from build123d import *

# Parameters (mm, degrees)
SKETCH_1_W               = 120
SKETCH_1_H               = 50
EXTRUDE_2_DEPTH          = 2.5
SKETCH_1_3_R             = 1.75
SKETCH_1_3_W             = 68
SKETCH_1_3_H             = 31
CUT_EXTRUDE_1_DEPTH      = 66.296266207
EXTRUDE_START            = -60
EXTRUDE_3_DEPTH          = 120
EXTRUDE_3_2_DEPTH        = 2.5
EXTRUDE_START_2          = 57.5
EXTRUDE_3_3_DEPTH        = 2.5
CUT_EXTRUDE_2_DEPTH      = 129.109700543
CUT_EXTRUDE_2_DEPTH_BACK = 129.109700543
EXTRUDE_4_DEPTH          = 120
EXTRUDE_5_REACH          = 77.063
EXTRUDE_6_REACH          = 77.063
SKETCH_7_R               = 2.5
CUT_EXTRUDE_3_DEPTH      = 5
SKETCH_8_R               = 1.75
CUT_EXTRUDE_4_DEPTH      = 5
EXTRUDE_8_DEPTH          = 120
SKETCH_10_W              = 3.2
SKETCH_10_H              = 2.2
CUT_EXTRUDE_5_DEPTH      = 10


# Read off the part's stored shape, not the designer's step: 凸台-拉伸3
with BuildPart() as part:
    # 草图1 → 凸台-拉伸2 (new, along a direction that is not the sketch's normal)
    with BuildSketch(Plane(origin=(0, 0, 0), x_dir=(1, 0, 0), z_dir=(0, 1, 0))):
        Rectangle(SKETCH_1_W, SKETCH_1_H)
    extrude(amount=EXTRUDE_2_DEPTH, dir=(0, 0.9659258262890672, 0.2588190451025249))

    # 草图1<3> → 切除-拉伸1 (cut, through all)
    with BuildSketch(Plane(origin=(0, 0, 0), x_dir=(1, 0, 0), z_dir=(0, 1, 0))):
        with Locations(Location((-45.5, 16.5, 0), (0, 0, 270))):
            Circle(SKETCH_1_3_R)
        with Locations(Location((-45.5, -16.5, 0), (0, 0, 270))):
            Circle(SKETCH_1_3_R)
        Rectangle(SKETCH_1_3_W, SKETCH_1_3_H)
        with BuildLine():
            Line((41.5, 18.25), (40.5, 18.25))
            ThreePointArc((40.5, 18.25), (38.75, 16.5), (40.5, 14.75))
            Line((40.5, 14.75), (41.5, 14.75))
            ThreePointArc((41.5, 14.75), (43.25, 16.5), (41.5, 18.25))
        make_face()
        with BuildLine():
            Line((41.5, -18.25), (40.5, -18.25))
            ThreePointArc((40.5, -18.25), (38.75, -16.5), (40.5, -14.75))
            Line((40.5, -14.75), (41.5, -14.75))
            ThreePointArc((41.5, -14.75), (43.25, -16.5), (41.5, -18.25))
        make_face()
    extrude(amount=CUT_EXTRUDE_1_DEPTH, mode=Mode.SUBTRACT)

    # 凸台-拉伸3 outline → 凸台-拉伸3 (add)
    with BuildSketch(Plane.YZ.offset(EXTRUDE_START)):
        Polygon((-10.306305876, -25.173375885), (-9.659258263, -27.588190451), (0, -25), (0, -22.411809549), align=None)
        Polygon((-25.188400969, 30.367359126), (-24.541353356, 27.952544561), (0, 34.528380374), (0, 37.116570825), align=None)
    extrude(amount=EXTRUDE_3_DEPTH)

    # Extrude 3 2 outline → Extrude 3 2 (add)
    with BuildSketch(Plane.YZ.offset(EXTRUDE_START)):
        Polygon((-24.541353356, 27.952544561), (-10.306305876, -25.173375885), (0, -22.411809549), (0, 34.528380374), align=None)
    extrude(amount=EXTRUDE_3_2_DEPTH)

    # Extrude 3 3 outline → Extrude 3 3 (add)
    with BuildSketch(Plane.YZ.offset(EXTRUDE_START_2)):
        Polygon((-24.541353356, 27.952544561), (-10.306305876, -25.173375885), (0, -22.411809549), (0, 34.528380374), align=None)
    extrude(amount=EXTRUDE_3_3_DEPTH)

    # 草图4 → 切除-拉伸2 (cut, two sides: drawn at the far end of the back side and taken through both)
    with BuildSketch(Plane.ZY.offset(60).offset(-CUT_EXTRUDE_2_DEPTH_BACK)):
        Polygon((25.647047613, 2.414814566), (36.951962095, -0.61432814), (37.116570825, 0), align=None)
    extrude(amount=CUT_EXTRUDE_2_DEPTH + CUT_EXTRUDE_2_DEPTH_BACK, mode=Mode.SUBTRACT)

    # 草图5 → 凸台-拉伸4 (add)
    with BuildSketch(Plane.ZY.offset(60)):
        Polygon((25.647047613, 2.414814566), (36.951962095, -0.61432814), (36.304914483, -3.029142706), (25, 0), align=None)
    extrude(amount=-EXTRUDE_4_DEPTH)

    # 凸台-拉伸5: up to this plane
    extrude_5_end = Plane(origin=(0, 0, 0), z_dir=(0, 1, 0))
    # 草图6 → 凸台-拉伸5 (add, up to the surface)
    with BuildSketch(Plane(origin=(0, -15.909258263, -4.262872904), x_dir=(1, 0, 0), z_dir=(0, -0.9659258262890672, -0.25881904510252496)), mode=Mode.PRIVATE) as extrude_5_sk1:
        with BuildLine():
            Line((-60, -24.148145657), (-52, -24.148145657))
            Line((-52, -24.148145657), (-52, -20.148145657))
            ThreePointArc((-52, -20.148145657), (-53.171572875, -17.319718532), (-56, -16.148145657))
            Line((-56, -16.148145657), (-60, -16.148145657))
            Line((-60, -16.148145657), (-60, -24.148145657))
        make_face()
    extrude_5_tool1 = split(extrude(extrude_5_sk1.sketch, amount=-EXTRUDE_5_REACH, mode=Mode.PRIVATE), bisect_by=extrude_5_end, keep=Keep.BOTH, mode=Mode.PRIVATE)
    add(extrude_5_tool1.solids().sort_by_distance((-56.176115, -10.648952, -23.894601))[0])
    # 草图6 → 凸台-拉伸5 (add, up to the surface)
    with BuildSketch(Plane(origin=(0, -15.909258263, -4.262872904), x_dir=(1, 0, 0), z_dir=(0, -0.9659258262890672, -0.25881904510252496)), mode=Mode.PRIVATE) as extrude_5_sk2:
        with BuildLine():
            Line((60, -24.148145657), (52, -24.148145657))
            Line((52, -24.148145657), (52, -20.148145657))
            ThreePointArc((52, -20.148145657), (53.171572875, -17.319718532), (56, -16.148145657))
            Line((56, -16.148145657), (60, -16.148145657))
            Line((60, -16.148145657), (60, -24.148145657))
        make_face()
    extrude_5_tool2 = split(extrude(extrude_5_sk2.sketch, amount=-EXTRUDE_5_REACH, mode=Mode.PRIVATE), bisect_by=extrude_5_end, keep=Keep.BOTH, mode=Mode.PRIVATE)
    add(extrude_5_tool2.solids().sort_by_distance((56.176115, -10.648952, -23.894601))[0])

    # 草图6<4> → 凸台-拉伸6 (add, up to next)
    with BuildSketch(Plane(origin=(0, -15.909258263, -4.262872904), x_dir=(1, 0, 0), z_dir=(0, -0.9659258262890672, -0.25881904510252496)), mode=Mode.PRIVATE) as extrude_6_sk1:
        with BuildLine():
            Line((-60, 35.851854343), (-52, 35.851854343))
            Line((-52, 35.851854343), (-52, 31.851854343))
            ThreePointArc((-52, 31.851854343), (-53.171572875, 29.023427218), (-56, 27.851854343))
            Line((-56, 27.851854343), (-60, 27.851854343))
            Line((-60, 27.851854343), (-60, 35.851854343))
        make_face()
    extrude_6_tool1 = extrude(extrude_6_sk1.sketch, amount=-EXTRUDE_6_REACH, mode=Mode.PRIVATE) - part.part
    # 草图6<4> → 凸台-拉伸6 (add, up to next)
    with BuildSketch(Plane(origin=(0, -15.909258263, -4.262872904), x_dir=(1, 0, 0), z_dir=(0, -0.9659258262890672, -0.25881904510252496)), mode=Mode.PRIVATE) as extrude_6_sk2:
        with BuildLine():
            Line((60, 35.851854343), (52, 35.851854343))
            Line((52, 35.851854343), (52, 31.851854343))
            ThreePointArc((52, 31.851854343), (53.171572875, 29.023427218), (56, 27.851854343))
            Line((56, 27.851854343), (60, 27.851854343))
            Line((60, 27.851854343), (60, 35.851854343))
        make_face()
    extrude_6_tool2 = extrude(extrude_6_sk2.sketch, amount=-EXTRUDE_6_REACH, mode=Mode.PRIVATE) - part.part
    add(extrude_6_tool1.solids().sort_by_distance((-56.176115, -24.198707, 26.67377))[0])
    add(extrude_6_tool2.solids().sort_by_distance((56.176115, -24.198707, 26.67377))[0])

    # 草图7 → 切除-拉伸3 (cut)
    with BuildSketch(Plane(origin=(0, -15.909258263, -4.262872904), x_dir=(1, 0, 0), z_dir=(0, -0.9659258262890672, -0.25881904510252496))):
        with Locations(Location((-56, 31.851854343, 0), (0, 0, 270))):
            Circle(SKETCH_7_R)
        with Locations(Location((-56, -20.148145657, 0), (0, 0, 270))):
            Circle(SKETCH_7_R)
        with Locations(Location((56, -20.148145657, 0), (0, 0, 270))):
            Circle(SKETCH_7_R)
        with Locations(Location((56, 31.851854343, 0), (0, 0, 270))):
            Circle(SKETCH_7_R)
    extrude(amount=-CUT_EXTRUDE_3_DEPTH, mode=Mode.SUBTRACT)

    # 草图8 → 切除-拉伸4 (cut)
    with BuildSketch(Plane(origin=(0, -11.079629131, -2.968777678), x_dir=(1, 0, 0), z_dir=(0, -0.9659258262890672, -0.25881904510252496))):
        with Locations(Location((-56, 31.851854343, 0), (0, 0, 270))):
            Circle(SKETCH_8_R)
        with Locations(Location((-56, -20.148145657, 0), (0, 0, 270))):
            Circle(SKETCH_8_R)
        with Locations(Location((56, -20.148145657, 0), (0, 0, 270))):
            Circle(SKETCH_8_R)
        with Locations(Location((56, 31.851854343, 0), (0, 0, 270))):
            Circle(SKETCH_8_R)
    extrude(amount=-CUT_EXTRUDE_4_DEPTH, mode=Mode.SUBTRACT)

    # 草图11 → 凸台-拉伸8 (add)
    with BuildSketch(Plane.ZY.offset(60)):
        Polygon((25.647047613, 2.414814566), (37.763618437, 2.414814566), (36.951962095, -0.61432814), align=None)
    extrude(amount=-EXTRUDE_8_DEPTH)

    # 草图10 → 切除-拉伸5 (cut)
    with BuildSketch(Plane(origin=(0, 6.25, 1.674682453), x_dir=(1, 0, 0), z_dir=(0, -0.9659258262890672, -0.25881904510252524))):
        with Locations((33.4, 29.251854343)):
            Rectangle(SKETCH_10_W, SKETCH_10_H)
        with Locations((43.4, 29.251854343)):
            Rectangle(SKETCH_10_W, SKETCH_10_H)
        with Locations((23.4, 29.251854343)):
            Rectangle(SKETCH_10_W, SKETCH_10_H)
    extrude(amount=-CUT_EXTRUDE_5_DEPTH, mode=Mode.SUBTRACT)


solid = part.part
Geometry check sheet. Reference: the model listing, model coordinates, mm. A direction names the side the tool comes from. Give positions to 0.01 mm unless a question says otherwise; leave off trailing zeros. Write each loop counter-clockwise with the first axis right and the second up, starting at its lowest first coordinate (ties: lowest second). Pieces come first, ordered by that corner, then holes.
1) Thickness scan on line 1 (X direction, y = 1.55, z = 16.5); line 2 (X direction, y = -10.25, z = -18.5); line 3 (Z direction, x = -45.5, y = 1.35). Record the ranges inside material, lowest first.
Values follow:
line 1: x = -60 to -47.25, -43.75 to 38.75, 43.25 to 60
line 2: x = -60 to -57.5, 57.5 to 60
line 3: z = -24.64 to -18.25, -14.75 to 14.75, 18.25 to 37.48
2) Cross-section at B-B (x = 46.5). Record the boundary of the cut face in (y, z).
Values follow:
outline: (-25.19, 30.37) - (-24.54, 27.95) - (-2.38, 33.89) - (0, 25) - (0, -22.41) - (-10.31, -25.17) - (-9.66, -27.59) - (2.41, -24.35) - (2.41, 37.76) - close
3) Go/stop test with flat-tipped pins: pin 1 Ø1.2 at (x, y) = (13, 1) entering from +Z; pin 2 Ø1.1 at (x, y) = (41, 2) entering from -Z; pin 3 Ø8 at (x, z) = (35, -14.5) entering from -Y; pin 4 Ø10 at (x, z) = (-15, 25.5) entering from -Y. Record where each tip stops, or that it passes through.
Values follow:
pin 1: stops at z = 37.55
pin 2: stops at z = -24.61
pin 3: stops at y = 0
pin 4: stops at y = -25.19
4) Cross-section at A-A (x = 0). Record the boundary of the cut face in (y, z).
Values follow:
outline: (-25.19, 30.37) - (-24.54, 27.95) - (-2.38, 33.89) - (0, 25) - (0, 15.5) - (2.41, 15.5) - (2.41, 37.76) - close; (-10.31, -25.17) - (-9.66, -27.59) - (2.41, -24.35) - (2.41, -15.5) - (0, -15.5) - (0, -22.41) - close
5) Set-up check for faces 3 (the face through (38.75, 1.19, -16.54)), 4 (the face through (-55.98, -14.5, 29.12)), 5 (the face through (-52, -5, -23)): record each of +Z, -Z, +X, -X, +Y, -Y from which the full face is reachable in a straight line by a thin tool's end or side.
Values follow:
face 3: +Y, -Y
face 4: none
face 5: -Y
6) Release check for a two-part mould opening along X. For faces 1 (the face through (-56.74, -12.19, 25.57)), 2 (the face through (-60, -8, 6)) record: released by +X, released by -X, zero draft, split by the parting line, or undercut.
Values follow:
face 1: undercut
face 2: released by -X
7) Cross-section at D-D (y = -21.5). Count the separate pieces of the cut face and the enclosed holes in it, plus the area to 3 significant figures.
Values follow:
separate pieces: 1
enclosed holes: 2
area: 386 mm2
8) Cross-section at C-C (z = 11.5). Record the boundary of the cut face in (x, y).
Values follow:
outline: (-60, -20.13) - (-57.5, -20.13) - (-57.5, 0) - (-34, 0) - (-34, 2.41) - (-60, 2.41) - close; (34, 0) - (57.5, 0) - (57.5, -20.13) - (60, -20.13) - (60, 2.41) - (34, 2.41) - close
